Model file for the job. Use its own axes, mm. A direction names the side the tool comes from. Coordinates: 2 decimals unless noted, no trailing zeros. Order: outer loops, then holes, each group sorted by start corner. A loop starts at its lowest first (then second) coordinate and runs counter-clockwise, first axis right, second up. Notation, with made-up numbers: M 75,55.5 L 93,55.5 A33 ccw 93,83.5 Z; hole C -6.75,8 d11. An arc over 180 degrees is marked long. Return JSON: item names as keys, results as strings.
```python
from build123d import *

# Parameters (mm, degrees)
BOSS_EXTRUDE1_DEPTH = 7
SKETCH3_W           = 40
SKETCH3_H           = 10
BOSS_EXTRUDE2_DEPTH = 50
SKETCH4_R           = 11
BOSS_EXTRUDE3_DEPTH = 7
SKETCH6_R           = 2.6
CUT_EXTRUDE1_DEPTH  = 7


with BuildPart() as part:
    # Sketch2 → Boss-Extrude1 (new body)
    with BuildSketch(Plane.XY):
        with BuildLine():
            Line((-20, 0), (-120, 0))
            ThreePointArc((-120, 0), (-134.142135624, 5.857864376), (-140, 20))
            Line((-140, 20), (-140, 40))
            ThreePointArc((-140, 40), (-134.142135624, 54.142135624), (-120, 60))
            Line((-120, 60), (-20, 60))
            ThreePointArc((-20, 60), (-5.857864376, 54.142135624), (0, 40))
            Line((0, 40), (0, 20))
            ThreePointArc((0, 20), (-5.857864376, 5.857864376), (-20, 0))
        make_face()
        with BuildLine():
            Line((-115, 50), (-25, 50))
            ThreePointArc((-25, 50), (-10.857864376, 44.142135624), (-5, 30))
            ThreePointArc((-5, 30), (-10.857864376, 15.857864376), (-25, 10))
            Line((-25, 10), (-115, 10))
            ThreePointArc((-115, 10), (-129.142135624, 15.857864376), (-135, 30))
            ThreePointArc((-135, 30), (-129.142135624, 44.142135624), (-115, 50))
        make_face(mode=Mode.SUBTRACT)
    extrude(amount=BOSS_EXTRUDE1_DEPTH)

    # Sketch3 → Boss-Extrude2 (add)
    with BuildSketch(Plane.XY.offset(7)):
        with Locations((-70, 55)):
            Rectangle(SKETCH3_W, SKETCH3_H)
        with Locations((-70, 5)):
            Rectangle(SKETCH3_W, SKETCH3_H)
    extrude(amount=BOSS_EXTRUDE2_DEPTH)

    # Sketch4 → Boss-Extrude3 (add)
    with BuildSketch(Plane.XY.offset(57)):
        with BuildLine():
            Line((-120, 60), (-20, 60))
            ThreePointArc((-20, 60), (-5.857864376, 54.142135624), (0, 40))
            Line((0, 40), (0, 20))
            ThreePointArc((0, 20), (-5.857864376, 5.857864376), (-20, 0))
            Line((-20, 0), (-120, 0))
            ThreePointArc((-120, 0), (-134.142135624, 5.857864376), (-140, 20))
            Line((-140, 20), (-140, 40))
            ThreePointArc((-140, 40), (-134.142135624, 54.142135624), (-120, 60))
        make_face()
        with Locations((-115.5, 30)):
            Circle(SKETCH4_R, mode=Mode.SUBTRACT)
        with Locations((-24.5, 30)):
            Circle(SKETCH4_R, mode=Mode.SUBTRACT)
    extrude(amount=BOSS_EXTRUDE3_DEPTH)

    # Sketch6 → Cut-Extrude1 (cut)
    with BuildSketch(Plane(origin=(0, 0, 0), x_dir=(-1, 0, 0), z_dir=(0, 0, -1))):
        with Locations((12.5, 50)):
            Circle(SKETCH6_R)
        with Locations((127.5, 50)):
            Circle(SKETCH6_R)
        with Locations((127.5, 10)):
            Circle(SKETCH6_R)
        with Locations((12.5, 10)):
            Circle(SKETCH6_R)
    extrude(amount=-CUT_EXTRUDE1_DEPTH, mode=Mode.SUBTRACT)


solid = part.part
```
Item 1: Saw through at C-C (z = 59.5). Write the cut outline in (x, y), and give its area (3 significant figures).
Check result:
{"outline": "M -140,20 A20 ccw -120,0 L -20,0 A20 ccw 0,20 L 0,40 A20 ccw -20,60 L -120,60 A20 ccw -140,40 Z; hole C -115.5,30 d22; hole C -24.5,30 d22", "area": "7,300 mm2"}
Item 2: Saw through at A-A (x = -94). Write the cut outline in (y, z), and give its area (3 significant figures).
Check result:
{"outline": "M 0,0 L 10,0 L 10,7 L 0,7 Z; M 0,57 L 60,57 L 60,64 L 0,64 Z; M 50,0 L 60,0 L 60,7 L 50,7 Z", "area": "560 mm2"}
Item 3: Pull direction Z, two halves, no side cores. Call faces 1 (the flat face through (-50, 5, 32)), 2 (the flat face through (-69, 30, 64)), 3 (the flat face through (0, 30, 3)): +Z half, -Z half, draft (parallel to the pull), parting line (faces both ways), or undercut.
Check result:
{"face 1": "undercut", "face 2": "+Z half", "face 3": "draft"}
Item 4: Drop flat-ended pins along their axis: pin 1 Ø1 at (y, z) = (53, 14) entering from -X; pin 2 Ø17.5 at (x, y) = (-24.5, 30) entering from -Z; pin 3 Ø11 at (y, z) = (53, 20.5) entering from +X; pin 4 Ø4 at (x, y) = (-12.5, 50) entering from -Z. Give the stop position or say it passes through.
Check result:
{"pin 1": "stops at x = -90", "pin 2": "passes through", "pin 3": "stops at x = -50", "pin 4": "stops at z = 57"}
Item 5: Saw through at B-B (z = 45). Write the cut outline in (x, y), and give its area (3 significant figures).
Check result:
{"outline": "M -90,0 L -50,0 L -50,10 L -90,10 Z; M -90,50 L -50,50 L -50,60 L -90,60 Z", "area": "800 mm2"}
Item 6: Saw through at D-D (x = -128). Write the cut outline in (y, z).
Check result:
{"outline": "M 1.67,0 L 7.45,0 L 7.45,7 L 1.67,7 Z; M 1.67,57 L 58.33,57 L 58.33,64 L 1.67,64 Z; M 12.55,0 L 14.8,0 L 14.8,7 L 12.55,7 Z; M 45.2,0 L 47.45,0 L 47.45,7 L 45.2,7 Z; M 52.55,0 L 58.33,0 L 58.33,7 L 52.55,7 Z"}
Item 7: Wall check: line 1 (Y direction, x = -24.5, z = 61.25); line 2 (Z direction, x = -119.5, y = 7); line 3 (Y direction, x = -127.5, z = 4.5). Give the ranges that are in metal, low to high.
Check result:
{"line 1": "y = 0 to 19, 41 to 60", "line 2": "z = 0 to 7, 57 to 64", "line 3": "y = 1.46 to 7.4, 12.6 to 14.39, 45.61 to 47.4, 52.6 to 58.54"}
Item 8: 3-axis set-ups, long thin cutter, end or side, ignore diameter. For faces 4 (the cylindrical face through (-134.297, 53.986, 60.451)), 5 (the flat face through (-131, 44, 7)), 6 (the flat face through (-50, 55, 32)), 7 (the flat face through (-71, 60, 32)), 8 (the flat face through (-69, 10, 28)): which of +Z, -Z, +X, -X, +Y, -Y reach the whole face in a straight line?
Check result:
{"face 4": "+Z, -Z, -X, +Y", "face 5": "-X, +Y, -Y", "face 6": "+X, +Y, -Y", "face 7": "+Z, -Z, +X, -X, +Y", "face 8": "-Z"}
